from build123d import *

# Parameters (mm, degrees)
F0_W         = 81.28
F0_H         = 82.804
F0_W_2       = 77.216
F0_H_2       = 78.74
F1_DEPTH     = 7.62
F2_DEPTH     = 1.524
F3_R         = 2.54
F4_R         = 1.27
F5_R         = 2.54
F6_DEPTH     = 25.4
F7_T1_DEPTH  = 20.32
F7_T4_ANGLE  = 90
F7_T6_ANGLE  = 90
F7_T8_ANGLE  = 90
F7_T10_ANGLE = 90


# Not quite as in the source:
# - a fillet or chamfer that OpenCascade refuses, or shapes differently, is made with other operations: its cross-section is extruded or revolved along the edge and cut away or added


with BuildPart() as f1:
    # F0 (on Top) → F1 (new body)
    with BuildSketch(Plane.XY):
        Rectangle(F0_W, F0_H)
        Rectangle(F0_W_2, F0_H_2, mode=Mode.SUBTRACT)
    extrude(amount=F1_DEPTH)

    # F0 (on Top) → F2 (join)
    with BuildSketch(Plane.XY):
        Rectangle(F0_W, F0_H)
        Rectangle(F0_W_2, F0_H_2, mode=Mode.SUBTRACT)
        Rectangle(F0_W_2, F0_H_2)
    extrude(amount=F2_DEPTH)

    # F3
    f3_edges = [f1.edges().sort_by_distance(p)[0] for p in [
        (-38.608, 39.37, 4.572),
        (38.608, 39.37, 4.572),
        (38.608, -39.37, 4.572),
        (-38.608, -39.37, 4.572),
        (0, 41.402, 0),
        (-40.64, 0, 0),
        (0, -41.402, 0),
        (40.64, 0, 0),
    ]]
    fillet(f3_edges, radius=F3_R)

    # F4
    f4_edges = [f1.edges().sort_by_distance(p)[0] for p in [
        (-38.608, 0, 1.524),
        (-37.864051, -38.626051, 1.524),
        (-37.864051, 38.626051, 1.524),
        (0, -39.37, 1.524),
        (0, 39.37, 1.524),
        (37.864051, -38.626051, 1.524),
        (37.864051, 38.626051, 1.524),
        (38.608, 0, 1.524),
    ]]
    fillet(f4_edges, radius=F4_R)

    # F5 (on face) → F6 (cut)
    with BuildSketch(Plane.XY.offset(1.524)):
        with Locations((0, 28.956)):
            Circle(F5_R)
        with Locations((0, 14.478)):
            Circle(F5_R)
        Circle(F5_R)
        with Locations((0, -14.478)):
            Circle(F5_R)
        with Locations((0, -28.956)):
            Circle(F5_R)
    extrude(amount=-F6_DEPTH, mode=Mode.SUBTRACT)

    # F7: fillet of radius 5.08 on 4 edges, made by hand

    # F7_s2 → F7_t1 (cut)
    with BuildSketch(Plane.XY):
        with BuildLine():
            ThreePointArc((35.56, -41.402), (39.1521024484, -39.9141024484), (40.64, -36.322))
            Line((40.64, -36.322), (40.64, -41.402))
            Line((40.64, -41.402), (35.56, -41.402))
        make_face()
        with BuildLine():
            ThreePointArc((35.56, 41.402), (39.1521024484, 39.9141024484), (40.64, 36.322))
            Line((40.64, 36.322), (40.64, 41.402))
            Line((40.64, 41.402), (35.56, 41.402))
        make_face()
        with BuildLine():
            ThreePointArc((-35.56, 41.402), (-39.1521024484, 39.9141024484), (-40.64, 36.322))
            Line((-40.64, 36.322), (-40.64, 41.402))
            Line((-40.64, 41.402), (-35.56, 41.402))
        make_face()
        with BuildLine():
            ThreePointArc((-40.64, -36.322), (-39.1521024484, -39.9141024484), (-35.56, -41.402))
            Line((-35.56, -41.402), (-40.64, -41.402))
            Line((-40.64, -41.402), (-40.64, -36.322))
        make_face()
    extrude(amount=F7_T1_DEPTH, mode=Mode.SUBTRACT)

    # F7_s3 → F7_t4 (revolve, cut)
    with BuildSketch(Plane.YZ.offset(-35.56)):
        with BuildLine():
            ThreePointArc((-38.862, 0), (-40.6580512242, 0.7439487758), (-41.402, 2.54))
            Line((-41.402, 2.54), (-41.402, 0))
            Line((-41.402, 0), (-38.862, 0))
        make_face()
    revolve(axis=Axis((-35.56, -36.322, 0), (0, 0, -1)), revolution_arc=F7_T4_ANGLE, mode=Mode.SUBTRACT)

    # F7_s5 → F7_t6 (revolve, cut)
    with BuildSketch(Plane.XZ.offset(-36.322)):
        with BuildLine():
            ThreePointArc((-38.1, 0), (-39.8960512242, 0.7439487758), (-40.64, 2.54))
            Line((-40.64, 2.54), (-40.64, 0))
            Line((-40.64, 0), (-38.1, 0))
        make_face()
    revolve(axis=Axis((-35.56, 36.322, 0), (0, 0, -1)), revolution_arc=F7_T6_ANGLE, mode=Mode.SUBTRACT)

    # F7_s7 → F7_t8 (revolve, cut)
    with BuildSketch(Plane.YZ.offset(35.56)):
        with BuildLine():
            ThreePointArc((38.862, 0), (40.6580512242, 0.7439487758), (41.402, 2.54))
            Line((41.402, 2.54), (41.402, 0))
            Line((41.402, 0), (38.862, 0))
        make_face()
    revolve(axis=Axis((35.56, 36.322, 0), (0, 0, -1)), revolution_arc=F7_T8_ANGLE, mode=Mode.SUBTRACT)

    # F7_s9 → F7_t10 (revolve, cut)
    with BuildSketch(Plane.XZ.offset(36.322)):
        with BuildLine():
            ThreePointArc((38.1, 0), (39.8960512242, 0.7439487758), (40.64, 2.54))
            Line((40.64, 2.54), (40.64, 0))
            Line((40.64, 0), (38.1, 0))
        make_face()
    revolve(axis=Axis((35.56, -36.322, 0), (0, 0, -1)), revolution_arc=F7_T10_ANGLE, mode=Mode.SUBTRACT)


solid = f1.part
Here's how the part is built. I have some questions about the finished solid (model axes, mm). A direction names the side the tool comes from. Coordinates: 2 decimals unless noted, no trailing zeros. Loops run counter-clockwise (first coordinate to the right, second up) from the corner with the lowest first, then second, coordinate; pieces in that order, holes last.
1. Imagine slicing it at B-B, the plane x = 0. Count the separate pieces of the cut face and the enclosed holes in it, and give its area (3 significant figures).
2. I need wall thicknesses on L1, parallel to X at y = 17, z = 5.25; L2, parallel to Y at x = -21.5, z = 6.75; L3, parallel to Y at x = 0, z = 0.3. Which ranges of each line are inside material? Lowest first, please.
3. For faces 4 (the cylindrical face through (-37.88, 38.61, 5.24)), 5 (the cylindrical face through (-39.916, 0.509, 0.764)), which set-ups out of +Z, -Z, +X, -X, +Y, -Y let a thin tool reach every point of the face, with its end or its side?
4. For P1, Ø1, axis at x = 27, z = 1.5, coming from the +Y side; P2, Ø8, axis at x = -3, y = -7.5, coming from the +Z side, each with a flat end and sliding along its axis, tell me the tip position at first contact or that it passes through.
5. If we mould it in two halves opening along Y, with no side actions, what happens to faces 1 (the cylindrical face through (-37.88, -38.61, 5.24)), 2 (the flat face through (-40.64, -1, 5)), 3 (the cylindrical face through (39.112, -39.953, 5.044))? For each: pulls with the +Y half, pulls with the -Y half, needs draft (parallel to the pull), parting line crosses it, or undercut.
6. Imagine slicing it at C-C, the plane y = -20.5. Please give me the cut outline in (x, z), and give its area (3 significant figures).
7. Imagine slicing it at A-A, the plane y = 0. Please give me the cut outline in (x, z), and give its area (3 significant figures).
Taken from the geometry:
1. separate pieces: 6
1. enclosed holes: 0
1. area: 110 mm2
2. L1: x = -40.64 to -38.61, 38.61 to 40.64
2. L2: y = -41.4 to -39.37, 39.37 to 41.4
2. L3: y = -40.06 to -31.5, -26.42 to -17.02, -11.94 to -2.54, 2.54 to 11.94, 17.02 to 26.42, 31.5 to 40.06
3. face 4: +Z
3. face 5: -Z, -X, +Y, -Y
4. P1: stops at y = 41.34
4. P2: stops at z = 1.52
5. face 1: undercut
5. face 2: needs draft
5. face 3: pulls with the -Y half
6. outline: (-40.64, 2.54) arc R2.54 ccw to (-38.1, 0) - (38.1, 0) arc R2.54 ccw to (40.64, 2.54) - (40.64, 7.62) - (38.61, 7.62) - (38.61, 2.79) arc R1.27 cw to (37.34, 1.52) - (-37.34, 1.52) arc R1.27 cw to (-38.61, 2.79) - (-38.61, 7.62) - (-40.64, 7.62) - close
6. area: 147 mm2
7. outline: (-40.64, 2.54) arc R2.54 ccw to (-38.1, 0) - (-2.54, 0) - (-2.54, 1.52) - (-37.34, 1.52) arc R1.27 cw to (-38.61, 2.79) - (-38.61, 7.62) - (-40.64, 7.62) - close; (2.54, 0) - (38.1, 0) arc R2.54 ccw to (40.64, 2.54) - (40.64, 7.62) - (38.61, 7.62) - (38.61, 2.79) arc R1.27 cw to (37.34, 1.52) - (2.54, 1.52) - close
7. area: 139 mm2
